```python
from build123d import *

# Parameters (mm, degrees)
CYLINDER_R           = 2.65
CYLINDER_DEPTH       = 2.6
CYLINDER_PITCH_ANGLE = 90
FILLET001_R          = 0.5
PAD001_DEPTH         = 0.4
FILLET002_R          = 0.25
SKETCH_W             = 12
SKETCH_H             = 12
PAD_DEPTH            = 6.5
FILLET_R             = 0.5


with BuildPart() as fillet001:
    # Cylinder → Cylinder (new body)
    with BuildSketch(Plane.XY):
        Circle(CYLINDER_R)
    extrude(amount=CYLINDER_DEPTH)


with BuildPart() as fillet001_1:
    # Cylinder pitch: moved
    add(fillet001.part.rotate(Axis((0, 0, 0), (0, 1, 0)), CYLINDER_PITCH_ANGLE))


with BuildPart() as fillet001_2:
    # Cylinder placement: moved
    add(fillet001_1.part.moved(Location((6.5, 0, 0))))

    # Fillet001
    fillet001_edges = [fillet001_2.edges().sort_by_distance(p)[0] for p in [
        (9.1, 0, 2.65),
    ]]
    fillet(fillet001_edges, radius=FILLET001_R)


with BuildPart() as fillet002:
    # Sketch001 → Pad001 (new body)
    with BuildSketch(Plane.YZ.offset(3.4)):
        Polygon((-3.25, -6), (-2.05, -6), (-2.05, -9), (-2.35, -10), (-2.35, -12), (-2.95, -12), (-2.95, -10), (-3.25, -9), align=None)
        Polygon((2.05, -6), (3.25, -6), (3.25, -9), (2.95, -10), (2.95, -12), (2.35, -12), (2.35, -10), (2.05, -9), align=None)
    extrude(amount=PAD001_DEPTH)

    # Fillet002
    fillet002_edges = [fillet002.edges().sort_by_distance(p)[0] for p in [
        (3.6, 2.95, -12),
        (3.6, 2.35, -12),
        (3.6, -2.35, -12),
        (3.6, -2.95, -12),
    ]]
    fillet(fillet002_edges, radius=FILLET002_R)


with BuildPart() as fusion:
    # Sketch → Pad (new body)
    with BuildSketch(Plane.YZ):
        Rectangle(SKETCH_W, SKETCH_H)
    extrude(amount=PAD_DEPTH)

    # Fillet
    fillet_edges = [fusion.edges().sort_by_distance(p)[0] for p in [
        (3.25, 6, 6),
        (3.25, -6, 6),
        (3.25, -6, -6),
        (3.25, 6, -6),
    ]]
    fillet(fillet_edges, radius=FILLET_R)

    # Fusion: union Fillet001, Fillet002
    add(fillet001_2.part)
    add(fillet002.part)


solid = fusion.part
```
The model under review builds one solid part; all positions refer to its coordinate system, in mm. A direction names the side the tool comes from. Round coordinates to 2 decimals unless told otherwise and drop trailing zeros. Write each loop counter-clockwise with the first axis right and the second up, starting at its lowest first coordinate (ties: lowest second). Pieces come first, ordered by that corner, then holes.
(1) We need section B-B on y = 0. Give the boundary of the cut face in (x, z), and give its area (3 significant figures).
(2) Machinability: for faces 1 (the cylindrical face through (7.54, -1.01, -2.45)), 2 (the flat face through (3.8, 3, -8)), 3 (the flat face through (3.4, -3, -8)), 4 (the flat face through (0, 0, 0)), which of the approach directions +Z, -Z, +X, -X, +Y, -Y give a long, thin tool a straight path to every point of the face, cutting with its end or side? Answer none if there is none.
(3) We need section A-A on x = 3. Give the boundary of the cut face in (y, z), and give its area (3 significant figures).
(4) Wall thickness on L1, parallel to Z at x = 6, y = 2.75; L2, parallel to Y at x = 3.5, z = -11; L3, parallel to X at y = 3.75, z = -1.5: over which ranges is each line inside the solid? List them lowest first.
(5) We need section C-C on z = -9.25. Give the boundary of the cut face in (x, y) (3 decimals).
(6) Insertion check: pin 1 (1 mm diameter, centred on y = 3, z = -9, fed in from +X); pin 2 (1 mm diameter, centred on x = 4.5, y = -3.5, fed in from -Z); pin 3 (0.6 mm diameter, centred on y = 2.5, z = -8.5, fed in from -X). Each pin has a flat end and moves straight along its axis. Give the tip position at first contact, or say it passes through.
Findings below:
1. outline: (0, -6) - (6.5, -6) - (6.5, -2.65) - (8.6, -2.65) arc R0.5 ccw to (9.1, -2.15) - (9.1, 2.15) arc R0.5 ccw to (8.6, 2.65) - (6.5, 2.65) - (6.5, 6) - (0, 6) - close
1. area: 91.7 mm2
2. face 1: +X
2. face 2: -Z, +X, +Y, -Y
2. face 3: -Z, -X, +Y, -Y
2. face 4: +Z, -Z, -X, +Y, -Y
3. outline: (-6, -5.5) arc R0.5 ccw to (-5.5, -6) - (5.5, -6) arc R0.5 ccw to (6, -5.5) - (6, 5.5) arc R0.5 ccw to (5.5, 6) - (-5.5, 6) arc R0.5 ccw to (-6, 5.5) - close
3. area: 144 mm2
4. L1: z = -6 to 6
4. L2: y = -2.95 to -2.35, 2.35 to 2.95
4. L3: x = 0 to 6.5
5. outline: (3.4, -3.175) - (3.8, -3.175) - (3.8, -2.125) - (3.4, -2.125) - close; (3.4, 2.125) - (3.8, 2.125) - (3.8, 3.175) - (3.4, 3.175) - close
6. pin 1: stops at x = 3.8
6. pin 2: stops at z = -6
6. pin 3: stops at x = 3.4
